Check sheet for the modelled part. Datum: model origin and axes. Units: mm. Give positions to 0.01 mm unless a question says otherwise; leave off trailing zeros. Write each loop counter-clockwise with the first axis right and the second up, starting at its lowest first coordinate (ties: lowest second). Pieces come first, ordered by that corner, then holes. Notation, with made-up numbers: (83.25, 34) -> (131.25, 34) arc R21 cw to (131.25, 44) -> close; hole circle Ø8 at (7.25, 6.25). An arc over 180 degrees is marked (long way). Answer as a JSON object with one key per item and string values.
from build123d import *

# Parameters (mm, degrees)
SKETCH1_W           = 70
SKETCH1_H           = 70
BOSS_EXTRUDE1_DEPTH = 2
SKETCH2_W           = 2
SKETCH2_H           = 20
SKETCH2_W_2         = 20
SKETCH2_H_2         = 2
CUT_EXTRUDE1_DEPTH  = 2
SKETCH3_W           = 6
SKETCH3_H           = 14
SKETCH3_W_2         = 7
SKETCH3_H_2         = 5
SKETCH3_H_3         = 6
SKETCH3_H_4         = 11
SKETCH3_H_5         = 9.678877381
SKETCH3_W_3         = 5.911764375
SKETCH3_W_4         = 8
SKETCH3_H_6         = 7
SKETCH3_H_7         = 11.067115318
SKETCH3_H_8         = 13.044819002
SKETCH3_W_5         = 12
CUT_EXTRUDE2_DEPTH  = 10


with BuildPart() as part:
    # Sketch1 → Boss-Extrude1 (new body)
    with BuildSketch(Plane.XY):
        Rectangle(SKETCH1_W, SKETCH1_H)
    extrude(amount=-BOSS_EXTRUDE1_DEPTH)

    # Sketch2 → Cut-Extrude1 (cut)
    with BuildSketch(Plane.XY):
        with Locations((-34, 15)):
            Rectangle(SKETCH2_W, SKETCH2_H)
        with Locations((-34, -15)):
            Rectangle(SKETCH2_W, SKETCH2_H)
        with Locations((-15, -34)):
            Rectangle(SKETCH2_W_2, SKETCH2_H_2)
        with Locations((15, -34)):
            Rectangle(SKETCH2_W_2, SKETCH2_H_2)
        with Locations((34, -15)):
            Rectangle(SKETCH2_W, SKETCH2_H)
        with Locations((34, 15)):
            Rectangle(SKETCH2_W, SKETCH2_H)
        with Locations((15, 34)):
            Rectangle(SKETCH2_W_2, SKETCH2_H_2)
        with Locations((-15, 34)):
            Rectangle(SKETCH2_W_2, SKETCH2_H_2)
    extrude(amount=-CUT_EXTRUDE1_DEPTH, mode=Mode.SUBTRACT)

    # Sketch3 → Cut-Extrude2 (cut)
    with BuildSketch(Plane.XY):
        with Locations((16.127037524, 11.743568931)):
            Rectangle(SKETCH3_W, SKETCH3_H)
        with Locations((9.627037524, 7.243568931)):
            Rectangle(SKETCH3_W_2, SKETCH3_H_2)
        with Locations((9.127037524, 19.5)):
            Rectangle(SKETCH3_W, SKETCH3_H_3)
        with Locations((12.681095539, -7.321122619)):
            Rectangle(SKETCH3_W, SKETCH3_H_4)
        with Locations((12.681095539, -17.66056131)):
            Rectangle(SKETCH3_W, SKETCH3_H_5)
        with Locations((18.636977726, -20)):
            Rectangle(SKETCH3_W_3, SKETCH3_H_2)
        with Locations((-14.154511362, -15.485830005)):
            Rectangle(SKETCH3_W_4, SKETCH3_H_6)
        with Locations((-3, -5.533557659)):
            Rectangle(SKETCH3_W, SKETCH3_H_7)
        with Locations((-3, 6.522409501)):
            Rectangle(SKETCH3_W, SKETCH3_H_8)
        with Locations((-12, 10.544819002)):
            Rectangle(SKETCH3_W_5, SKETCH3_H_2)
    extrude(amount=-CUT_EXTRUDE2_DEPTH, mode=Mode.SUBTRACT)


solid = part.part
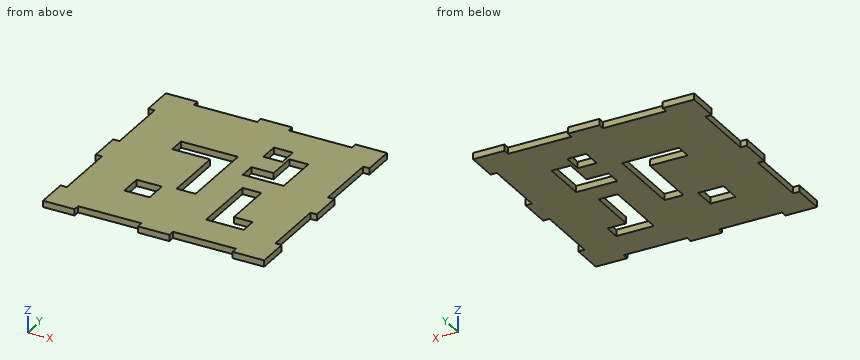
1. Sectioned sample at A-A, the plane y = 0.5. Enter the section's corners in (x, z).
Determined:
{"outline": "(-35, -2) -> (-6, -2) -> (-6, 0) -> (-35, 0) -> close; (0, -2) -> (35, -2) -> (35, 0) -> (0, 0) -> close"}
2. Sectioned sample at B-B, the plane x = 16.5. Enter the section's corners in (y, z), plus the area to 3 significant figures.
Determined:
{"outline": "(-33, -2) -> (-22.5, -2) -> (-22.5, 0) -> (-33, 0) -> close; (-17.5, -2) -> (4.74, -2) -> (4.74, 0) -> (-17.5, 0) -> close; (18.74, -2) -> (33, -2) -> (33, 0) -> (18.74, 0) -> close", "area": "94.0 mm^2"}
3. Sectioned sample at C-C, the plane y = -7.5. Enter the section's corners in (x, z).
Determined:
{"outline": "(-33, -2) -> (-6, -2) -> (-6, 0) -> (-33, 0) -> close; (0, -2) -> (9.68, -2) -> (9.68, 0) -> (0, 0) -> close; (15.68, -2) -> (33, -2) -> (33, 0) -> (15.68, 0) -> close"}
4. Go/stop test with flat-tipped pins: P1, Ø1, axis at x = 11.5, z = -1.5, coming from the -Y side; P2, Ø0.6, axis at y = -10, z = -1, coming from the +X side; P3, Ø0.6, axis at x = -15, z = -0.5, coming from the +Y side. Record where each tip stops, or that it passes through.
Determined:
{"P1": "y = -33", "P2": "x = 33", "P3": "y = 33"}
5. Scan lines: L1, parallel to X at y = 6, z = -1; L2, parallel to X at y = -9.5, z = -0.45; L3, parallel to Y at x = -13, z = -0.7. Record each from-to range of solid material in increasing order. Write a range as [from, to].
Determined:
{"L1": "[-33, -6], [0, 6.13], [19.13, 33]", "L2": "[-33, -6], [0, 9.68], [15.68, 33]", "L3": "[-33, -18.99], [-11.99, 8.04], [13.04, 33]"}
6. Sectioned sample at D-D, the plane y = -20.5. Enter the section's corners in (x, z), plus the area to 3 significant figures.
Determined:
{"outline": "(-33, -2) -> (9.68, -2) -> (9.68, 0) -> (-33, 0) -> close; (21.59, -2) -> (33, -2) -> (33, 0) -> (21.59, 0) -> close", "area": "108 mm^2"}
